from build123d import *

# Parameters (mm, degrees)
BOSS_EXTRUDE1_DEPTH = 48.42
BOSS_EXTRUDE2_DEPTH = 2.54
BOSS_EXTRUDE3_DEPTH = 2.54
FILLET1_R           = 3


with BuildPart() as part:
    # Sketch2 → Boss-Extrude1 (new body)
    with BuildSketch(Plane.XY):
        with BuildLine():
            Line((0, 5), (0, 74.46))
            ThreePointArc((0, 74.46), (0.816699867, 77.198612788), (3, 79.042575695))
            ThreePointArc((3, 79.042575695), (5.183300133, 77.198612788), (6, 74.46))
            Line((6, 74.46), (6, 11))
            ThreePointArc((6, 11), (7.464466094, 7.464466094), (11, 6))
            Line((11, 6), (27.877424305, 6))
            ThreePointArc((27.877424305, 6), (30.616037093, 5.183300133), (32.46, 3))
            ThreePointArc((32.46, 3), (30.616037093, 0.816699867), (27.877424305, 0))
            Line((27.877424305, 0), (6, 0))
            Line((6, 0), (5, 0))
            ThreePointArc((5, 0), (1.464466094, 1.464466094), (0, 5))
        make_face()
    extrude(amount=BOSS_EXTRUDE1_DEPTH)

    # Sketch3 → Boss-Extrude2 (add)
    with BuildSketch(Plane.XY.offset(48.42)):
        Polygon((-2.54, 81.582575695), (8.54, 81.582575695), (8.54, 8.54), (35, 8.54), (35, -2.54), (-2.54, -2.54), align=None)
    extrude(amount=BOSS_EXTRUDE2_DEPTH)

    # Sketch4 → Boss-Extrude3 (add)
    with BuildSketch(Plane(origin=(0, 0, 0), x_dir=(-1, 0, 0), z_dir=(0, 0, -1))):
        Polygon((-35, -2.54), (2.54, -2.54), (2.54, 81.582575695), (-8.54, 81.582575695), (-8.54, 8.54), (-35, 8.54), align=None)
    extrude(amount=BOSS_EXTRUDE3_DEPTH)

    # Fillet1
    fillet1_edges = [part.edges().sort_by_distance(p)[0] for p in [
        (-2.54, 81.582575695, 49.69),
        (-2.54, -2.54, 49.69),
        (35, -2.54, 49.69),
        (35, 8.54, 49.69),
        (8.54, 8.54, 49.69),
        (8.54, 81.582575695, 49.69),
        (35, 8.54, -1.27),
        (35, -2.54, -1.27),
        (-2.54, -2.54, -1.27),
        (-2.54, 81.582575695, -1.27),
        (8.54, 81.582575695, -1.27),
        (8.54, 8.54, -1.27),
    ]]
    fillet(fillet1_edges, radius=FILLET1_R)


solid = part.part
Could you check a few things on this model? Use its own coordinates, in mm. A direction names the side the tool comes from. Round coordinates to 2 decimals unless told otherwise and drop trailing zeros. Order: outer loops, then holes, each group sorted by start corner. A loop starts at its lowest first (then second) coordinate and runs counter-clockwise, first axis right, second up.
Q1. I'm going to push flat-ended pins straight in: P1, Ø1, axis at y = 51.5, z = 42.5, coming from the +X side; P2, Ø1.3, axis at y = 42, z = -2, coming from the +X side; P3, Ø1.3, axis at x = 19.5, z = 49.5, coming from the +Y side. Where does each tip first touch, or does it pass through?
Geometry says:
P1: stops at x = 6
P2: stops at x = 8.54
P3: stops at y = 8.54
Q2. Thinking about a two-plate mould opening in Z: for faces 1 (the face through (22, 8.54, 50)), 2 (the face through (19, 6, 24)), 3 (the face through (8, 31, 50.96)), which applies, released by +Z, released by -Z, zero draft, split by the parting line, or undercut?
Geometry says:
face 1: zero draft
face 2: undercut
face 3: released by +Z
Q3. Imagine slicing it at A-A, the plane y = 48. List the corners of the cut face in (x, z) for me, then the cut area to 3 significant figures.
Geometry says:
outline: (-2.54, -2.54) - (8.54, -2.54) - (8.54, 0) - (6, 0) - (6, 48.42) - (8.54, 48.42) - (8.54, 50.96) - (-2.54, 50.96) - (-2.54, 48.42) - (0, 48.42) - (0, 0) - (-2.54, 0) - close
area: 347 mm2
Q4. Please list where these lines run through material, in increasing order: probe 1 along Z at (x, y) = (-1, 28.5); probe 2 along Y at (x, z) = (16.5, 4.5).
Geometry says:
probe 1: z = -2.54 to 0, 48.42 to 50.96
probe 2: y = 0 to 6
Q5. Which directions (+Z, -Z, +X, -X, +Y, -Y) give clear straight access to the entire face, cutting with the end or side of a thin tool? Please do faces 4 (the face through (22, 8.54, -1)), 5 (the face through (30.65, 0.84, 23.87)), 6 (the face through (30.582, 5.205, 23.871)), 7 (the face through (7, 33, 0)).
Geometry says:
face 4: +Z, -Z, +X, +Y
face 5: +X, -Y
face 6: +X, +Y
face 7: none
Q6. Imagine slicing it at C-C, the plane z = 42.5. List the corners of the cut face in (x, y) for me, then the cut area to 3 significant figures.
Geometry says:
outline: (0, 5) arc R5 ccw to (5, 0) - (27.88, 0) arc R5 ccw to (32.46, 3) arc R5 ccw to (27.88, 6) - (11, 6) arc R5 cw to (6, 11) - (6, 74.46) arc R5 ccw to (3, 79.04) arc R5 ccw to (0, 74.46) - close
area: 618 mm2
